```python
from build123d import *

# Parameters (mm, degrees)
SKETCH1_R           = 69.85
SKETCH1_R_2         = 3.937
SKETCH1_R_3         = 6.35
SKETCH1_R_4         = 10.668
BOSS_EXTRUDE1_DEPTH = 3.175
SKETCH2_R           = 1.5875
CUT_EXTRUDE2_DEPTH  = 10
SKETCH2_4_R         = 1.5875
CUT_EXTRUDE3_DEPTH  = 10
BOSS_EXTRUDE3_START = 2.54
SKETCH2_5_W         = 6.35
SKETCH2_5_H         = 6.35
SKETCH2_5_R         = 1.5875
BOSS_EXTRUDE3_DEPTH = 2.54
SKETCH4_R           = 1.5
CUT_EXTRUDE4_DEPTH  = 6.35
BOSS_EXTRUDE4_START = 2.54
SKETCH4_4_W         = 6.35
SKETCH4_4_H         = 6.35
SKETCH4_4_R         = 1.5
BOSS_EXTRUDE4_DEPTH = 2.54


with BuildPart() as part:
    # Sketch1 → Boss-Extrude1 (new body)
    with BuildSketch(Plane(origin=(0, 0, 0), x_dir=(1, 0, 0), z_dir=(0, 1, 0))):
        with Locations(Location((0, 0, 0), (0, 0, 270))):
            Circle(SKETCH1_R)
        with Locations(Location((-51.795490029, -24.152633658, 0), (0, 0, 270))):
            Circle(SKETCH1_R_2, mode=Mode.SUBTRACT)
        with Locations(Location((-53.975, 0, 0), (0, 0, 270))):
            Circle(SKETCH1_R_3, mode=Mode.SUBTRACT)
        with Locations(Location((-50.64447914, 23.615908466, 0), (0, 0, 270))):
            Circle(SKETCH1_R_4, mode=Mode.SUBTRACT)
        with Locations(Location((51.795490029, 24.152633658, 0), (0, 0, 270))):
            Circle(SKETCH1_R_2, mode=Mode.SUBTRACT)
        with Locations(Location((53.975, 0, 0), (0, 0, 270))):
            Circle(SKETCH1_R_3, mode=Mode.SUBTRACT)
        with Locations(Location((50.64447914, -23.615908466, 0), (0, 0, 270))):
            Circle(SKETCH1_R_4, mode=Mode.SUBTRACT)
    extrude(amount=BOSS_EXTRUDE1_DEPTH)

    # Sketch2 → Cut-Extrude2 (cut)
    with BuildSketch(Plane(origin=(0, 3.175, 0), x_dir=(1, 0, 0), z_dir=(0, 1, 0))):
        with Locations(Location((-28.575, -28.575, 0), (0, 0, 270))):
            Circle(SKETCH2_R)
    extrude(amount=-CUT_EXTRUDE2_DEPTH, mode=Mode.SUBTRACT)

    # Sketch2_4 → Cut-Extrude3 (cut)
    with BuildSketch(Plane(origin=(0, 3.175, 0), x_dir=(1, 0, 0), z_dir=(0, 1, 0))):
        with Locations(Location((-28.575, 28.575, 0), (0, 0, 270))):
            Circle(SKETCH2_4_R)
        with Locations(Location((28.575, 28.575, 0), (0, 0, 270))):
            Circle(SKETCH2_4_R)
        with Locations(Location((28.575, -28.575, 0), (0, 0, 270))):
            Circle(SKETCH2_4_R)
    extrude(amount=-CUT_EXTRUDE3_DEPTH, mode=Mode.SUBTRACT)

    # Sketch2_5 → Boss-Extrude3 (add)
    # profile 1 of 4: a face of its own
    with BuildSketch(Plane(origin=(0, 3.175, 0), x_dir=(1, 0, 0), z_dir=(0, 1, 0)).offset(BOSS_EXTRUDE3_START)):
        with Locations((-28.575, 28.575)):
            Rectangle(SKETCH2_5_W, SKETCH2_5_H)
        with Locations(Location((-28.575, 28.575, 0), (0, 0, 270))):
            Circle(SKETCH2_5_R, mode=Mode.SUBTRACT)
    # profile 2 of 4: a face of its own
    with BuildSketch(Plane(origin=(0, 3.175, 0), x_dir=(1, 0, 0), z_dir=(0, 1, 0)).offset(BOSS_EXTRUDE3_START)):
        with Locations((28.575, 28.575)):
            Rectangle(SKETCH2_5_W, SKETCH2_5_H)
        with Locations(Location((28.575, 28.575, 0), (0, 0, 270))):
            Circle(SKETCH2_5_R, mode=Mode.SUBTRACT)
    # profile 3 of 4: a face of its own
    with BuildSketch(Plane(origin=(0, 3.175, 0), x_dir=(1, 0, 0), z_dir=(0, 1, 0)).offset(BOSS_EXTRUDE3_START)):
        with Locations((-28.575, -28.575)):
            Rectangle(SKETCH2_5_W, SKETCH2_5_H)
        with Locations(Location((-28.575, -28.575, 0), (0, 0, 270))):
            Circle(SKETCH2_5_R, mode=Mode.SUBTRACT)
    # profile 4 of 4: a face of its own
    with BuildSketch(Plane(origin=(0, 3.175, 0), x_dir=(1, 0, 0), z_dir=(0, 1, 0)).offset(BOSS_EXTRUDE3_START)):
        with Locations((28.575, -28.575)):
            Rectangle(SKETCH2_5_W, SKETCH2_5_H)
        with Locations(Location((28.575, -28.575, 0), (0, 0, 270))):
            Circle(SKETCH2_5_R, mode=Mode.SUBTRACT)
    extrude(amount=-BOSS_EXTRUDE3_DEPTH)

    # Sketch4 → Cut-Extrude4 (cut)
    with BuildSketch(Plane(origin=(0, 3.175, 0), x_dir=(1, 0, 0), z_dir=(0, 1, 0))):
        with Locations(Location((10.235820896, 55.249992322, 0), (0, 0, 270))):
            Circle(SKETCH4_R)
        with Locations(Location((-18.847179104, 41.279992322, 0), (0, 0, 270))):
            Circle(SKETCH4_R)
    extrude(amount=-CUT_EXTRUDE4_DEPTH, mode=Mode.SUBTRACT)

    # Sketch4_4 → Boss-Extrude4 (add)
    # profile 1 of 2: a face of its own
    with BuildSketch(Plane(origin=(0, 3.175, 0), x_dir=(1, 0, 0), z_dir=(0, 1, 0)).offset(BOSS_EXTRUDE4_START)):
        with Locations((-18.847179104, 41.279992322)):
            Rectangle(SKETCH4_4_W, SKETCH4_4_H)
        with Locations(Location((-18.847179104, 41.279992322, 0), (0, 0, 270))):
            Circle(SKETCH4_4_R, mode=Mode.SUBTRACT)
    # profile 2 of 2: a face of its own
    with BuildSketch(Plane(origin=(0, 3.175, 0), x_dir=(1, 0, 0), z_dir=(0, 1, 0)).offset(BOSS_EXTRUDE4_START)):
        with Locations((10.235820896, 55.249992322)):
            Rectangle(SKETCH4_4_W, SKETCH4_4_H)
        with Locations(Location((10.235820896, 55.249992322, 0), (0, 0, 270))):
            Circle(SKETCH4_4_R, mode=Mode.SUBTRACT)
    extrude(amount=-BOSS_EXTRUDE4_DEPTH)


solid = part.part
```
Design review of the part built by this model. Coordinates are the model's own, in mm. Give positions to 0.01 mm unless a question says otherwise; leave off trailing zeros. Write each loop counter-clockwise with the first axis right and the second up, starting at its lowest first coordinate (ties: lowest second). Pieces come first, ordered by that corner, then holes.
(1) Add section A-A (z = 0). Give the boundary of the cut face in (x, y) (3 decimals), and give its area (3 significant figures).
Checked values:
outline: (-69.85, 0) - (-60.325, 0) - (-60.325, 3.175) - (-69.85, 3.175) - close; (-47.625, 0) - (47.625, 0) - (47.625, 3.175) - (-47.625, 3.175) - close; (60.325, 0) - (69.85, 0) - (69.85, 3.175) - (60.325, 3.175) - close
area: 363 mm2
(2) Clearance check with flat-ended pins moving along their axes: pin 1 Ø3 at (x, y) = (-43.5, 2) entering from -Z; pin 2 Ø1.3 at (y, z) = (4.5, -27) entering from -X; pin 3 Ø3 at (y, z) = (4, -41) entering from -X; pin 4 Ø13 at (x, z) = (50.64, 23.62) entering from -Y. State where each tip first meets the part, or that it passes through.
Checked values:
pin 1: stops at z = -55.81
pin 2: stops at x = -31.75
pin 3: stops at x = -57.44
pin 4: passes through
(3) Add section C-C (y = 1.55). Give the number of separate pieces and of enclosed holes in the cut face, and give its area (3 significant figures).
Checked values:
separate pieces: 1
enclosed holes: 12
area: 14,200 mm2
(4) Wall thickness on line 1 along X through (y, z) = (1.15, 0) (3 decimals); line 2 along X through (y, z) = (3.35, 26); line 3 along X through (y, z) = (0.4, -26): over which ranges is each line inside the solid? List them lowest first.
Checked values:
line 1: x = -69.85 to -60.325, -47.625 to 47.625, 60.325 to 69.85
line 2: x = -31.75 to -25.4, 25.4 to 31.75
line 3: x = -64.83 to -61.04, -40.25 to 48.32, 55.27 to 64.83
(5) Mouldability with a two-part tool opening along X and no side actions: class faces 1 (the face through (-68.2, 1.6, -15.1)), 2 (the face through (12, 5.715, -55)), 3 (the face through (-27.502, 2.898, 27.405)) as +X half, -X half, draft (parallel to the pull), parting line (faces both ways), or undercut.
Checked values:
face 1: parting line
face 2: draft
face 3: undercut
(6) Add section B-B (x = -43.5). Give the boundary of the cut face in (y, z) (3 decimals).
Checked values:
outline: (0, -54.651) - (3.175, -54.651) - (3.175, -31.538) - (0, -31.538) - close; (0, -15.694) - (3.175, -15.694) - (3.175, 54.651) - (0, 54.651) - close
(7) Add section D-D (x = 0). Give the boundary of the cut face in (y, z) (3 decimals).
Checked values:
outline: (0, -69.85) - (3.175, -69.85) - (3.175, 69.85) - (0, 69.85) - close
